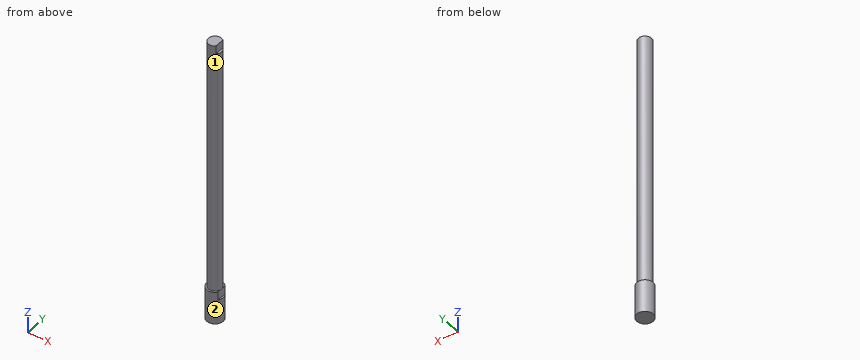
Solid Edge part; units mm, degrees
sketch "Sketch1" plane through (0, 0, 0) normal (0, 0, 1) x (1, 0, 0)
  circle A0 centre (0, 0) radius 5
extrude "Protrusion1" add sketch "Sketch1" along normal blind 20
sketch "Sketch2" plane through (0, 0, 20) normal (0, 0, 1) x (1, 0, 0)
  circle A0 centre (0, 0) radius 4
extrude "ExtrudedProtrusion_2" add sketch "Sketch2" along normal blind 155
sketch "Sketch3" plane through (0, 0, 20) normal (0, 0, 1) x (0, -1, 0)
  line L0 (-3.8216, 6.2347) -> (3.8216, 6.2347)
  line L1 (3.8216, 6.2347) -> (3.8216, 4)
  line L2 (3.8216, 4) -> (0, 4)
  line L3 (0, 4) -> (-3.8216, 4)
  line L4 (-3.8216, 4) -> (-3.8216, 6.2347)
extrude "ExtrudedCutout_1" cut sketch "Sketch3" against normal blind 5
sketch "Sketch4" plane through (0, 0, 175) normal (0, 0, 1) x (0, -1, 0)
  line L0 (-3.2306, 4) -> (4.2507, 4)
  line L1 (4.2507, 4) -> (4.2507, 2.6458)
  line L2 (4.2507, 2.6458) -> (0, 2.6458)
  line L3 (0, 2.6458) -> (-3.2306, 2.6458)
  line L4 (-3.2306, 2.6458) -> (-3.2306, 4)
extrude "ExtrudedCutout_2" cut sketch "Sketch4" against normal blind 5
Source: CAD feature listing. Evaluate the final solid. Frame: model axes, mm. Face numbers are marked on the shaded views. A direction names the side the tool comes from. Round coordinates to 2 decimals unless told otherwise and drop trailing zeros. Loops run counter-clockwise (first coordinate to the right, second up) from the corner with the lowest first, then second, coordinate; pieces in that order, holes last.
(1) Access query for the marked faces 1 and 2. Directions: +Z, -Z, +X, -X, +Y, -Y. A direction counts if a zero-diameter tool reaches every point of the face in a straight line with its end or side. Return the directions, or none.
From the geometry:
face 1: +Z
face 2: +Z, -Z
(2) Section query A-A (x = 0). Output: boundary loops of the cut face in (y, z), and give its area (3 significant figures).
From the geometry:
outline: (-5, 0) - (5, 0) - (5, 20) - (4, 20) - (4, 175) - (-4, 175) - (-4, 20) - (-5, 20) - close
area: 1,440 mm2
(3) Material intervals for probe 1 along Z at (x, y) = (-3.75, 1.5); probe 2 along X at (y, z) = (0.5, 59.5); probe 3 along X at (y, z) = (2.25, 96.5), sorted ascending.
From the geometry:
probe 1: z = 0 to 20
probe 2: x = -3.97 to 3.97
probe 3: x = -3.31 to 3.31
(4) Section query B-B (z = 37). Output: boundary loops of the cut face in (x, y).
From the geometry:
outline: circle Ø8 at (0, 0)
(5) Contact query for flat-ended pins moving along their axis: pin 1 Ø2 at (y, z) = (-1.5, 32) entering from -X; pin 2 Ø1 at (x, z) = (1.5, 36) entering from -Y; pin 3 Ø1.5 at (y, z) = (1, 171.5) entering from +X. Output: stop coordinate, or through.
From the geometry:
pin 1: stops at x = -3.97
pin 2: stops at y = -3.87
pin 3: stops at x = 2.65
